For this review, take the finished solid that the model builds, in its own axes (mm). Face numbers are marked on the shaded views. Give positions to 0.01 mm unless a question says otherwise; leave off trailing zeros. Loops run counter-clockwise (first coordinate to the right, second up) from the corner with the lowest first, then second, coordinate; pieces in that order, holes last. Notation, with made-up numbers: (74.25, 51.5) - (122.25, 51.5) arc R24 cw to (122.25, 75.5) - close; hole circle Ø7 at (25.5, 49.5). An arc over 180 degrees is marked (long way). Answer in a Markdown table with one row per item.
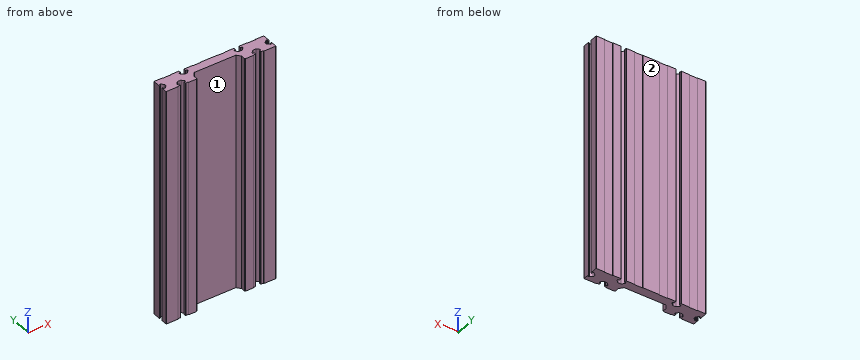
```python
from build123d import *

# Parameters (mm, degrees)
Y_KSEKLIK_EKSTR_ZYON1_DEPTH = 300


with BuildPart() as part:
    # Çizim1 → Yükseklik-Ekstrüzyon1 (new body)
    with BuildSketch(Plane.XY):
        with BuildLine():
            Line((0.5, 0), (15.3, 0))
            Line((15.3, 0), (15.3, 0.75))
            Line((15.3, 0.75), (18.5, 0.75))
            Line((18.5, 0.75), (18.8, 1.05))
            Line((18.8, 1.05), (18.8, 3.25))
            Line((18.8, 3.25), (16.8, 3.25))
            Line((16.8, 3.25), (16.8, 4.542893219))
            ThreePointArc((16.8, 4.542893219), (16.838060234, 4.734234935), (16.946446609, 4.896446609))
            Line((16.946446609, 4.896446609), (19.401845417, 7.351845417))
            ThreePointArc((19.401845417, 7.351845417), (19.969586278, 7.731197732), (20.639282284, 7.86440855))
            Line((20.639282284, 7.86440855), (23.360717716, 7.86440855))
            ThreePointArc((23.360717716, 7.86440855), (24.030413722, 7.731197732), (24.598154583, 7.351845417))
            Line((24.598154583, 7.351845417), (27.053553391, 4.896446609))
            ThreePointArc((27.053553391, 4.896446609), (27.161939766, 4.734234935), (27.2, 4.542893219))
            Line((27.2, 4.542893219), (27.2, 3.25))
            Line((27.2, 3.25), (25.2, 3.25))
            Line((25.2, 3.25), (25.2, 1.05))
            Line((25.2, 1.05), (25.5, 0.75))
            Line((25.5, 0.75), (28.7, 0.75))
            Line((28.7, 0.75), (28.7, 0))
            Line((28.7, 0), (38.882330038, 0))
            Line((38.882330038, 0), (39.482330038, 0.6))
            Line((39.482330038, 0.6), (39.482330038, 6.1))
            Line((39.482330038, 6.1), (43.5, 10.888072611))
            Line((43.5, 10.888072611), (96.5, 10.888072611))
            Line((96.5, 10.888072611), (100.517669962, 6.1))
            Line((100.517669962, 6.1), (100.517669962, 0.6))
            Line((100.517669962, 0.6), (101.117669962, 0))
            Line((101.117669962, 0), (111.3, 0))
            Line((111.3, 0), (111.3, 0.75))
            Line((111.3, 0.75), (114.5, 0.75))
            Line((114.5, 0.75), (114.8, 1.05))
            Line((114.8, 1.05), (114.8, 3.25))
            Line((114.8, 3.25), (112.8, 3.25))
            Line((112.8, 3.25), (112.8, 4.542893219))
            ThreePointArc((112.8, 4.542893219), (112.838060234, 4.734234935), (112.946446609, 4.896446609))
            Line((112.946446609, 4.896446609), (115.401845417, 7.351845417))
            ThreePointArc((115.401845417, 7.351845417), (115.969586278, 7.731197732), (116.639282284, 7.86440855))
            Line((116.639282284, 7.86440855), (119.360717716, 7.86440855))
            ThreePointArc((119.360717716, 7.86440855), (120.030413722, 7.731197732), (120.598154583, 7.351845417))
            Line((120.598154583, 7.351845417), (123.053553391, 4.896446609))
            ThreePointArc((123.053553391, 4.896446609), (123.161939766, 4.734234935), (123.2, 4.542893219))
            Line((123.2, 4.542893219), (123.2, 3.25))
            Line((123.2, 3.25), (121.2, 3.25))
            Line((121.2, 3.25), (121.2, 1.05))
            Line((121.2, 1.05), (121.5, 0.75))
            Line((121.5, 0.75), (124.7, 0.75))
            Line((124.7, 0.75), (124.7, 0))
            Line((124.7, 0), (139.5, 0))
            ThreePointArc((139.5, 0), (139.853553391, 0.146446609), (140, 0.5))
            Line((140, 0.5), (140, 7.8))
            Line((140, 7.8), (138.75, 7.8))
            Line((138.75, 7.8), (138.75, 5.8))
            Line((138.75, 5.8), (137.431985117, 5.8))
            ThreePointArc((137.431985117, 5.8), (137.260975045, 5.83015369), (137.110591312, 5.916977778))
            Line((137.110591312, 5.916977778), (134.625121683, 8.002534428))
            ThreePointArc((134.625121683, 8.002534428), (134.163961373, 8.603530245), (134, 9.343112203))
            Line((134, 9.343112203), (134, 10.698544282))
            ThreePointArc((134, 10.698544282), (134.163961373, 11.43812624), (134.625121683, 12.039122058))
            Line((134.625121683, 12.039122058), (137.110591312, 14.124678707))
            ThreePointArc((137.110591312, 14.124678707), (137.260975045, 14.211502796), (137.431985117, 14.241656485))
            Line((137.431985117, 14.241656485), (138.75, 14.241656485))
            Line((138.75, 14.241656485), (138.75, 12.241656485))
            Line((138.75, 12.241656485), (140, 12.241656485))
            Line((140, 12.241656485), (140, 21.5))
            ThreePointArc((140, 21.5), (139.853553391, 21.853553391), (139.5, 22))
            Line((139.5, 22), (129.4, 22))
            Line((129.4, 22), (129.4, 21.5))
            Line((129.4, 21.5), (118.8, 21.5))
            Line((118.8, 21.5), (118.8, 22))
            Line((118.8, 22), (108.5, 22))
            Line((108.5, 22), (108.2, 21.7))
            Line((108.2, 21.7), (108.2, 19))
            Line((108.2, 19), (110.2, 19))
            Line((110.2, 19), (110.2, 17.707106781))
            ThreePointArc((110.2, 17.707106781), (110.161939766, 17.515765065), (110.053553391, 17.353553391))
            Line((110.053553391, 17.353553391), (107.598154583, 14.898154583))
            ThreePointArc((107.598154583, 14.898154583), (107.030413722, 14.518802268), (106.360717716, 14.38559145))
            Line((106.360717716, 14.38559145), (103.639282284, 14.38559145))
            ThreePointArc((103.639282284, 14.38559145), (102.969586278, 14.518802268), (102.401845417, 14.898154583))
            Line((102.401845417, 14.898154583), (99.946446609, 17.353553391))
            ThreePointArc((99.946446609, 17.353553391), (99.86234478, 17.525824053), (99.8, 17.707106781))
            Line((99.8, 17.707106781), (99.8, 19))
            Line((99.8, 19), (101.8, 19))
            Line((101.8, 19), (101.8, 21.7))
            Line((101.8, 21.7), (101.5, 22))
            Line((101.5, 22), (91.2, 22))
            Line((91.2, 22), (91.2, 21.5))
            Line((91.2, 21.5), (80.6, 21.5))
            Line((80.6, 21.5), (80.6, 22))
            Line((80.6, 22), (59.4, 22))
            Line((59.4, 22), (59.4, 21.5))
            Line((59.4, 21.5), (48.8, 21.5))
            Line((48.8, 21.5), (48.8, 22))
            Line((48.8, 22), (38.5, 22))
            Line((38.5, 22), (38.2, 21.7))
            Line((38.2, 21.7), (38.2, 19))
            Line((38.2, 19), (40.2, 19))
            Line((40.2, 19), (40.2, 17.707106781))
            ThreePointArc((40.2, 17.707106781), (40.13765522, 17.525824053), (40.053553391, 17.353553391))
            Line((40.053553391, 17.353553391), (37.598154583, 14.898154583))
            ThreePointArc((37.598154583, 14.898154583), (37.030413722, 14.518802268), (36.360717716, 14.38559145))
            Line((36.360717716, 14.38559145), (33.639282284, 14.38559145))
            ThreePointArc((33.639282284, 14.38559145), (32.969586278, 14.518802268), (32.401845417, 14.898154583))
            Line((32.401845417, 14.898154583), (29.946446609, 17.353553391))
            ThreePointArc((29.946446609, 17.353553391), (29.838060234, 17.515765065), (29.8, 17.707106781))
            Line((29.8, 17.707106781), (29.8, 19))
            Line((29.8, 19), (31.8, 19))
            Line((31.8, 19), (31.8, 21.7))
            Line((31.8, 21.7), (31.5, 22))
            Line((31.5, 22), (21.2, 22))
            Line((21.2, 22), (21.2, 21.5))
            Line((21.2, 21.5), (10.6, 21.5))
            Line((10.6, 21.5), (10.6, 22))
            Line((10.6, 22), (0.5, 22))
            ThreePointArc((0.5, 22), (0.146446609, 21.853553391), (0, 21.5))
            Line((0, 21.5), (0, 12.241656485))
            Line((0, 12.241656485), (1.25, 12.241656485))
            Line((1.25, 12.241656485), (1.25, 14.241656485))
            Line((1.25, 14.241656485), (2.568014883, 14.241656485))
            ThreePointArc((2.568014883, 14.241656485), (2.739024955, 14.211502796), (2.889408688, 14.124678707))
            Line((2.889408688, 14.124678707), (5.374878317, 12.039122058))
            ThreePointArc((5.374878317, 12.039122058), (5.836038627, 11.43812624), (6, 10.698544282))
            Line((6, 10.698544282), (6, 9.343112203))
            ThreePointArc((6, 9.343112203), (5.836038627, 8.603530245), (5.374878317, 8.002534428))
            Line((5.374878317, 8.002534428), (2.889408688, 5.916977778))
            ThreePointArc((2.889408688, 5.916977778), (2.739024955, 5.83015369), (2.568014883, 5.8))
            Line((2.568014883, 5.8), (1.25, 5.8))
            Line((1.25, 5.8), (1.25, 7.8))
            Line((1.25, 7.8), (0, 7.8))
            Line((0, 7.8), (0, 0.5))
            ThreePointArc((0, 0.5), (0.146446609, 0.146446609), (0.5, 0))
        make_face()
    extrude(amount=Y_KSEKLIK_EKSTR_ZYON1_DEPTH)


solid = part.part
```
1. Wall thickness on line 1 (X direction, y = 2, z = 124); line 2 (X direction, y = 3.5, z = 14); line 3 (X direction, y = 21.25, z = 260.5): over which ranges is each line inside the solid? List them lowest first. Write a range as [from, to].
Values:
| item | result |
|---|---|
| line 1 | x = [0, 18.8], [25.2, 39.48], [100.52, 114.8], [121.2, 140] |
| line 2 | x = [0, 16.8], [27.2, 39.48], [100.52, 112.8], [123.2, 140] |
| line 3 | x = [0, 31.8], [38.2, 101.8], [108.2, 140] |
2. Clearance check with flat-ended pins moving along their axes: pin 1 (1.4 mm diameter, centred on x = 105, z = 121.5, fed in from +Y); pin 2 (1 mm diameter, centred on x = 42.5, z = 113.5, fed in from -Y). State where each tip first meets the part, or that it passes through.
Values:
| item | result |
|---|---|
| pin 1 | stops at y = 14.39 |
| pin 2 | stops at y = 9.1 |
3. Mouldability with a two-part tool opening along X and no side actions: class the marked faces 1 and 2 as released by +X, released by -X, zero draft, split by the parting line, or undercut.
Values:
| item | result |
|---|---|
| face 1 | undercut |
| face 2 | zero draft |
4. We need section A-A, the plane x = 56. Give the boundary of the cut face in (y, z), and give its area (3 significant figures).
Values:
| item | result |
|---|---|
| outline | (10.89, 0) - (21.5, 0) - (21.5, 300) - (10.89, 300) - close |
| area | 3,180 mm^2 |
